Design review of the part built by this model. Coordinates are the model's own, in mm. A direction names the side the tool comes from. Coordinates: 2 decimals unless noted, no trailing zeros. Order: outer loops, then holes, each group sorted by start corner. A loop starts at its lowest first (then second) coordinate and runs counter-clockwise, first axis right, second up. Notation, with made-up numbers: (-16.75, -7.5) -> (11.25, -7.5) arc R17 cw to (11.25, 21.5) -> close; hole circle Ø5 at (1.5, 7). An arc over 180 degrees is marked (long way). Use a Markdown table: item, result. Add a question column.
Q1. Add section B-B (x = 0). State the section outline as (y, z) points, then the cut area to 3 significant figures.
Q2. Add section D-D (y = 3). State the section outline as (x, z) points.
Q3. Wall thickness on probe 1 along X at (y, z) = (4.5, -1); probe 2 along Z at (x, y) = (-5, 3); probe 3 along Z at (x, y) = (-4, 3.25): over which ranges is each line inside the solid? List them lowest first.
Q4. Insertion check: pin 1 (3 mm diameter, centred on y = 8, z = 14, fed in from -X); pin 2 (4.5 mm diameter, centred on x = 0, z = 13, fed in from -Y); pin 3 (3 mm diameter, centred on x = 13, z = 0, fed in from -Y); pin 4 (2 mm diameter, centred on x = -8, y = 3, fed in from -Z). Each pin has a flat end and moves straight along its axis. Give the tip position at first contact, or say it passes through.
Q5. The part is to be moulded in two halves that separate along Z. For faces 3 (the face through (15.747, 4.563, -8.191)), 4 (the face through (4, 9, -4)), 5 (the face through (0.526, 3.6, -11.331)), say which applies: pulls with the +Z half, pulls with the -Z half, needs draft (parallel to the pull), parting line crosses it, or undercut.
Q6. Machinability: for faces 1 (the face through (-8, 0, 8)), 2 (the face through (10.74, 3.45, 2.38)), which of the approach directions +Z, -Z, +X, -X, +Y, -Y give a long, thin tool a straight path to every point of the face, cutting with its end or side? Answer none if there is none.
Q7. Add section C-C (x = 13). State the section outline as (y, z) points.
Q8. Add section A-A (z = 0). State the section outline as (x, y) points.
from build123d import *

# Parameters (mm, degrees)
SKETCH4_R          = 1.75
CUT_EXTRUDE1_DEPTH = 9
CHAMFER1_SIZE      = 1.2
CHAMFER1_SIZE2     = 1.9


with BuildPart() as part:
    # Sketch3 → Revolve1 (revolve)
    with BuildSketch(Plane.XY, mode=Mode.PRIVATE) as revolve1_sk:
        Polygon((-11, 0), (-17.75, 0), (-17.75, 9), (-4.25, 9), (-4.25, 7), (-11, 7), align=None)
    revolve(revolve1_sk.sketch.rotate(Axis((0, 0, 0), (0, 1, 0)), 270), axis=Axis((0, 0, 0), (0, 1, 0)))

    # Sketch4 → Cut-Extrude1 (cut)
    with BuildSketch(Plane(origin=(0, 9, 0), x_dir=(1, 0, 0), z_dir=(0, 1, 0))):
        with Locations(Location((0, 13, 0), (0, 0, 270))):
            Circle(SKETCH4_R)
        with Locations(Location((13, 0, 0), (0, 0, 270))):
            Circle(SKETCH4_R)
        with Locations(Location((0, -13, 0), (0, 0, 270))):
            Circle(SKETCH4_R)
        with Locations(Location((-13, 0, 0), (0, 0, 270))):
            Circle(SKETCH4_R)
    extrude(amount=-CUT_EXTRUDE1_DEPTH, mode=Mode.SUBTRACT)

    # Chamfer1
    chamfer1_edges = [part.edges().sort_by_distance(p)[0] for p in [
        (0, 9, -14.75),
        (13, 9, -1.75),
        (0, 9, 11.25),
        (-13, 9, -1.75),
    ]]
    chamfer1_side = [part.faces().sort_by_distance(p)[0] for p in [
        (0, 9, 17.247954185),
    ]]
    chamfer(chamfer1_edges, length=CHAMFER1_SIZE, length2=CHAMFER1_SIZE2, reference=chamfer1_side[0])


solid = part.part
Established:
| question | item | result |
|---|---|---|
| 1 | outline | (0, -17.75) -> (9, -17.75) -> (9, -15.95) -> (7.1, -14.75) -> (0, -14.75) -> close; (0, -11.25) -> (7.1, -11.25) -> (9, -10.05) -> (9, -4.25) -> (7, -4.25) -> (7, -11) -> (0, -11) -> close; (0, 11) -> (7, 11) -> (7, 4.25) -> (9, 4.25) -> (9, 10.05) -> (7.1, 11.25) -> (0, 11.25) -> close; (0, 14.75) -> (7.1, 14.75) -> (9, 15.95) -> (9, 17.75) -> (0, 17.75) -> close |
| 1 | area | 80.9 mm^2 |
| 2 | outline | circle Ø35.5 at (0, 0); hole circle Ø3.5 at (-13, 0); hole circle Ø22 at (0, 0); hole circle Ø3.5 at (0, -13); hole circle Ø3.5 at (0, 13); hole circle Ø3.5 at (13, 0) |
| 3 | probe 1 | -17.72 to -14.44, -11.56 to -10.95, 10.95 to 11.56, 14.44 to 17.72 |
| 3 | probe 2 | -17.03 to -9.8, 9.8 to 17.03 |
| 3 | probe 3 | -17.29 to -10.25, 10.25 to 17.29 |
| 4 | pin 1 | x = -12.6 |
| 4 | pin 2 | y = 0 |
| 4 | pin 3 | through |
| 4 | pin 4 | z = -16.31 |
| 5 | face 3 | parting line crosses it |
| 5 | face 4 | needs draft |
| 5 | face 5 | undercut |
| 6 | face 1 | +Z, -Z, +X, -X, -Y |
| 6 | face 2 | -Y |
| 7 | outline | (0, -12.09) -> (9, -12.09) -> (9, -2.95) -> (7.1, -1.75) -> (0, -1.75) -> close; (0, 1.75) -> (7.1, 1.75) -> (9, 2.95) -> (9, 12.09) -> (0, 12.09) -> close |
| 8 | outline | (-17.75, 0) -> (-14.75, 0) -> (-14.75, 7.1) -> (-15.95, 9) -> (-17.75, 9) -> close; (-11.25, 0) -> (-11, 0) -> (-11, 7) -> (-4.25, 7) -> (-4.25, 9) -> (-10.05, 9) -> (-11.25, 7.1) -> close; (4.25, 7) -> (11, 7) -> (11, 0) -> (11.25, 0) -> (11.25, 7.1) -> (10.05, 9) -> (4.25, 9) -> close; (14.75, 0) -> (17.75, 0) -> (17.75, 9) -> (15.95, 9) -> (14.75, 7.1) -> close |
